Part model, mm, in its own coordinate system. A direction names the side the tool comes from. Give positions to 0.01 mm unless a question says otherwise; leave off trailing zeros. Loops run counter-clockwise (first coordinate to the right, second up) from the corner with the lowest first, then second, coordinate; pieces in that order, holes last. Notation, with made-up numbers: (37, 44.5) -> (65, 44.5) arc R24 ccw to (65, 82.5) -> close; hole circle Ø7 at (3.25, 66). An arc over 180 degrees is marked (long way). One line per question, with ' | ' between items.
```python
from build123d import *

# Parameters (mm, degrees)
BOSS_EXTRU_1_DEPTH = 5


with BuildPart() as part:
    # Esquisse1 → Boss.-Extru.1 (new body)
    with BuildSketch(Plane(origin=(0, 0, 0), x_dir=(1, 0, 0), z_dir=(0, 1, 0))):
        with BuildLine():
            Line((-85.986477301, -39.220909897), (-82.836538311, -36.274742561))
            ThreePointArc((-82.836538311, -36.274742561), (-84.826589539, -30.099452785), (-86.244619049, -23.768283856))
            ThreePointArc((-86.244619049, -23.768283856), (-86.563047935, -19.917311272), (-86.17049139, -16.073187685))
            ThreePointArc((-86.17049139, -16.073187685), (-78.973775537, 19.793847734), (-54.666943907, 47.13273734))
            ThreePointArc((-54.666943907, 47.13273734), (-53.551106318, 48.285581279), (-52.350511604, 49.349872124))
            ThreePointArc((-52.350511604, 49.349872124), (-61.160452612, 47.314883556), (-68.670306383, 42.279177512))
            ThreePointArc((-68.670306383, 42.279177512), (-89.686895205, 4.154921869), (-85.986477301, -39.220909897))
        make_face()
    extrude(amount=BOSS_EXTRU_1_DEPTH)


solid = part.part
```
1) Drill centre lines: line 1 (X direction, y = 4.75, z = 18); line 2 (Z direction, x = -80, y = 3.7); line 3 (Z direction, x = -77.5, y = 2.2). Where is each one in solid material? Low to high.
Found:
line 1: -91.04 to -86.46 | line 2: -28.2 to -17.64 | line 3: -31.96 to -22.59
2) Saw through at C-C (z = -24.5). Give the cut face in (x, y), and give its area (3 significant figures).
Found:
outline: (-82.16, 0) -> (-76.4, 0) -> (-76.4, 5) -> (-82.16, 5) -> close | area: 28.8 mm2
3) Saw through at A-A (y = 0.95). Give the cut face in (x, z).
Found:
outline: (-86.24, 23.77) arc R71 cw to (-82.84, 36.27) -> (-85.99, 39.22) arc R75 ccw to (-68.67, -42.28) arc R25 ccw to (-52.35, -49.35) arc R21 cw to (-54.67, -47.13) arc R70 cw to (-86.17, 16.07) arc R21 cw to start
4) Saw through at B-B (x = -69.5). Give the cut face in (y, z), and give its area (3 significant figures).
Found:
outline: (0, -41.46) -> (5, -41.46) -> (5, -34.09) -> (0, -34.09) -> close | area: 36.8 mm2
5) Pull direction Z, two halves, no side cores. Call faces 1 (the cylindrical face through (-86.563, 2.465, 19.971)), 2 (the flat face through (-84.434, 2.465, 37.768)), 3 (the flat face through (-83, 0, -12)), 4 (the cylindrical face through (-89.556, 2.465, -4.759)): pulls with the +Z half, pulls with the -Z half, needs draft (parallel to the pull), parting line crosses it, or undercut.
Found:
face 1: undercut | face 2: pulls with the +Z half | face 3: needs draft | face 4: parting line crosses it
6) Pin check, flat tips, straight feed: P1, Ø3, axis at y = 2, z = 27, coming from the -X side; P2, Ø2, axis at y = 1, z = 28.5, coming from the -X side; P3, Ø2, axis at x = -67.5, y = 3.5, coming from the +Z side. Stop position of each tip, or through.
Found:
P1: x = -89.99 | P2: x = -89.58 | P3: z = -35.23
7) Tool access for faces 5 (the cylindrical face through (-53.57, 2.46, -48.27)), 6 (the cylindrical face through (-84.8, 2.5, 30.2)): list every direction of +Z, -Z, +X, -X, +Y, -Y with a clear straight run to the whole face (end or side of a thin tool).
Found:
face 5: +Z, +X, +Y, -Y | face 6: +X, +Y, -Y
